```python
from build123d import *

# Parameters (mm, degrees)
F0_W     = 93.103454
F0_H     = 72.931036
F0_W_2   = 88.836216
F0_H_2   = 67.500002
F1_DEPTH = 5
F0_W_3   = 83.793112
F0_H_3   = 62.844828
F2_DEPTH = 1
F3_DEPTH = 4.6


with BuildPart() as f1:
    # F0 (on Top) → F1 (new body, symmetric)
    with BuildSketch(Plane.XY):
        Rectangle(F0_W, F0_H)
        Rectangle(F0_W_2, F0_H_2, mode=Mode.SUBTRACT)
    extrude(amount=F1_DEPTH, both=True)

    # F0 (on Top) → F2 (join)
    with BuildSketch(Plane.XY):
        Rectangle(F0_W_2, F0_H_2)
        Rectangle(F0_W_3, F0_H_3, mode=Mode.SUBTRACT)
    extrude(amount=F2_DEPTH)

    # F0 (on Top) → F3 (join)
    with BuildSketch(Plane.XY):
        Rectangle(F0_W_3, F0_H_3)
    extrude(amount=F3_DEPTH)


solid = f1.part
```
Geometry check sheet. Reference: the model listing, model coordinates, mm. A direction names the side the tool comes from. Round coordinates to 2 decimals unless told otherwise and drop trailing zeros. Loops run counter-clockwise (first coordinate to the right, second up) from the corner with the lowest first, then second, coordinate; pieces in that order, holes last. Notation, with made-up numbers: (10, -28.5) - (25, -28.5) arc R16 cw to (25, -6.5) - close; hole circle Ø8 at (21, 53.25). An arc over 180 degrees is marked (long way). Use a Markdown table: item, result.
Q1. Access from +Z, -Z, +X, -X, +Y, -Y to the whole of each face (thin tool, end or side, straight path). Record for faces 4 (the flat face through (-1, 33.75, 3)), 5 (the flat face through (-4, -35, -5)), 6 (the flat face through (-1, -33.75, -2)).
Solutions:
| item | result |
|---|---|
| face 4 | +Z |
| face 5 | -Z, +X, -X, +Y, -Y |
| face 6 | -Z |
Q2. Material ranges on line 1 (Y direction, x = 24.5, z = 2.75); line 2 (X direction, y = -29.5, z = 3.75); line 3 (X direction, y = -6, z = -4.25), recorded low to high.
Solutions:
| item | result |
|---|---|
| line 1 | y = -36.47 to -33.75, -31.42 to 31.42, 33.75 to 36.47 |
| line 2 | x = -46.55 to -44.42, -41.9 to 41.9, 44.42 to 46.55 |
| line 3 | x = -46.55 to -44.42, 44.42 to 46.55 |
Q3. Cross-section at B-B on y = -21. Record the cut outline in (x, z), plus the area to 3 significant figures.
Solutions:
| item | result |
|---|---|
| outline | (-46.55, -5) - (-44.42, -5) - (-44.42, 0) - (44.42, 0) - (44.42, -5) - (46.55, -5) - (46.55, 5) - (44.42, 5) - (44.42, 1) - (41.9, 1) - (41.9, 4.6) - (-41.9, 4.6) - (-41.9, 1) - (-44.42, 1) - (-44.42, 5) - (-46.55, 5) - close |
| area | 433 mm2 |
Q4. Cross-section at A-A on z = 2.25. Record the cut outline in (x, y), plus the area to 3 significant figures.
Solutions:
| item | result |
|---|---|
| outline | (-46.55, -36.47) - (46.55, -36.47) - (46.55, 36.47) - (-46.55, 36.47) - close; (-41.9, -31.42) - (41.9, -31.42) - (41.9, 31.42) - (-41.9, 31.42) - close; hole (-44.42, -33.75) - (44.42, -33.75) - (44.42, 33.75) - (-44.42, 33.75) - close |
| area | 6,060 mm2 |
Q5. Go/stop test with flat-tipped pins: P1, Ø1, axis at x = -14, y = -22, coming from the +Z side; P2, Ø6, axis at x = 18, y = -4, coming from the -Z side. Record where each tip stops, or that it passes through.
Solutions:
| item | result |
|---|---|
| P1 | stops at z = 4.6 |
| P2 | stops at z = 0 |
Q6. Draft check along X on faces 1 (the flat face through (-44.418, 0, -2)), 2 (the flat face through (46.552, -1, 0)), 3 (the flat face through (-4, -35, 5)). Enter one of: released by +X, released by -X, zero draft, split by the parting line, or undercut.
Solutions:
| item | result |
|---|---|
| face 1 | undercut |
| face 2 | released by +X |
| face 3 | zero draft |
Q7. Cross-section at C-C on x = -9. Record the cut outline in (y, z).
Solutions:
| item | result |
|---|---|
| outline | (-36.47, -5) - (-33.75, -5) - (-33.75, 0) - (33.75, 0) - (33.75, -5) - (36.47, -5) - (36.47, 5) - (33.75, 5) - (33.75, 1) - (31.42, 1) - (31.42, 4.6) - (-31.42, 4.6) - (-31.42, 1) - (-33.75, 1) - (-33.75, 5) - (-36.47, 5) - close |
